For this review, take the finished solid that the model builds, in its own axes (mm). A direction names the side the tool comes from. Give positions to 0.01 mm unless a question says otherwise; leave off trailing zeros. Order: outer loops, then holes, each group sorted by start corner. A loop starts at its lowest first (then second) coordinate and runs counter-clockwise, first axis right, second up.
Autodesk Fusion 360 part; units mm, degrees
sketch "Sketch1" plane through (0, 0, 0) normal (0, 0, 1) x (1, 0, 0)
  line L0 (4, 0) -> (4, 18)
  line L1 (4, 18) -> (9, 18)
  line L2 (9, 18) -> (9, 39)
  line L3 (9, 39) -> (5, 39)
  line L4 (5, 39) -> (5, 22)
  line L5 (5, 22) -> (-5, 22)
  line L6 (-5, 22) -> (-5, 39)
  line L7 (-5, 39) -> (-9, 39)
  line L8 (-9, 39) -> (-9, 18)
  line L9 (-9, 18) -> (-4, 18)
  line L10 (-4, 18) -> (-4, 0)
  line L11 (-4, 0) -> (4, 0)
  point P0 (0, 22)
  dimension "d1" = 10
  dimension "d2" = 17
  dimension "d3" = 4
  dimension "d4" = 18
  dimension "d5" = 4
  dimension "d6" = 8
extrude "Extrude1" add sketch "Sketch1" along normal blind 15
sketch "Sketch2" plane through (-9, 0, 0) normal (-1, 0, 0) x (0, -1, 0)
  line L0 (-39, 0) -> (-18, 0)
  line L1 (-18, 0) -> (-18, 15)
  line L2 (-18, 15) -> (-39, 15)
  line L3 (-39, 15) -> (-39, 0)
  circle A0 centre (-32, 7.5) radius 1.6
  line L4 (-22, 0) -> (-22, 15)
  line L5 (-8.8, 11.1) -> (-5, 11.1)
  line L6 (-5, 11.1) -> (-5, 3.9)
  line L7 (-5, 3.9) -> (-8.8, 3.9)
  line L8 (-8.8, 3.9) -> (-8.8, 11.1)
  line L9 (-8.8, 11.1) -> (-5, 3.9) construction
  line L10 (-5, 11.1) -> (-8.8, 3.9) construction
  line L11 (0, 0) -> (0, 15)
  point P0 (-39, 7.5)
  point P1 (-6.9, 7.5)
  point P2 (0, 7.5)
  dimension "d9" = 3.2
  dimension "d11" = 10
  dimension "d18" = 7.2
  dimension "d19" = 3.8
  dimension "d20" = 5
extrude "Extrude2" cut sketch "Sketch2" against normal up to surface (18 mm away) contours A0 | L5 L6 L7 L8
ref_plane "WorkPlane1" through (0, 19.5, 7.5) normal (0, 0, 1) x (1, 0, 0)
sketch "Sketch4" plane through (0, 17, 7.5) normal (0, 0, 1) x (1, 0, 0)
  line L0 (-5, 16.6) -> (-5, 13.4)
  line L1 (-9, 13.4) -> (-9, 16.6)
  line L2 (9, 16.6) -> (9, 13.4)
  line L3 (5, 13.4) -> (5, 16.6)
  line L4 (-9, 15) -> (9, 15) construction
  line L5 (-5, 13.4) -> (-5, 11.9)
  line L6 (-5, 11.9) -> (-4.25, 12.9)
  line L7 (-4.25, 12.9) -> (-4.25, 13.4)
  line L8 (-4.25, 13.4) -> (-5, 13.4)
  line L9 (5, 13.4) -> (5, 11.9)
  line L10 (5, 11.9) -> (4.25, 12.9)
  line L11 (4.25, 12.9) -> (4.25, 13.4)
  line L12 (4.25, 13.4) -> (5, 13.4)
  dimension "d14" = 0.75
  dimension "d15" = 0.5
  dimension "d16" = 1.5
revolve "Revolve1" add sketch "Sketch4" angle 360 about axis through (-9, 32, 7.5) along (1, 0, 0)
sketch "Sketch5" plane through (0, 0, 0) normal (0, -1, 0) x (1, 0, 0)
  line L0 (-4, 0) -> (4, 0)
  line L1 (4, 0) -> (4, 15)
  line L2 (4, 15) -> (-4, 15)
  line L3 (-4, 15) -> (-4, 0)
  circle A0 centre (0, 7.5) radius 2.1
  point P0 (-4, 7.5)
  dimension "d21" = 4.2
extrude "Extrude3" cut sketch "Sketch5" against normal blind 19 contours A0
fillet "Fillet1" radius 3 4 edges at (-9, 18, 7.5) (-9, 39, 7.5) (9, 39, 7.5) (9, 18, 7.5)
chamfer "Chamfer1" distance 1 angle 45 4 edges at (0, 0, 15) (-4, 0, 7.5) (0, 0, 0) (4, 0, 7.5)
sketch "Sketch6" plane through (-9, 0, 0) normal (-1, 0, 0) x (0, -1, 0)
  circle A0 centre (-32, 7.5) radius 1.6
  line L0 (-36, 15) -> (-36, 0)
  line L1 (-36, 0) -> (-21, 0)
  line L2 (-21, 0) -> (-21, 15)
  line L3 (-21, 15) -> (-36, 15)
  line L4 (-33.6454, 10.35) -> (-35.2909, 7.5)
  line L5 (-35.2909, 7.5) -> (-33.6454, 4.65)
  line L6 (-33.6454, 4.65) -> (-30.3546, 4.65)
  line L7 (-30.3546, 4.65) -> (-28.7091, 7.5)
  line L8 (-28.7091, 7.5) -> (-30.3546, 10.35)
  line L9 (-30.3546, 10.35) -> (-33.6454, 10.35)
  point P0 (-32, 7.5)
  dimension "d50" = 5.7
extrude "Extrude4" cut sketch "Sketch6" against normal blind 2 contours L4 L5 L6 L7 L8 L9
sketch "Sketch7" plane through (9, 0, 0) normal (1, 0, 0) x (0, 1, 0)
  circle A0 centre (32, 7.5) radius 1.6
  line L0 (21, 15) -> (21, 0)
  line L1 (21, 0) -> (36, 0)
  line L2 (36, 0) -> (36, 15)
  line L3 (36, 15) -> (21, 15)
  circle A1 centre (32, 7.5) radius 3
  dimension "d53" = 6
extrude "Extrude5" cut sketch "Sketch7" against normal blind 2 contours A1
1) Draft analysis for pull direction Y (two halves, no side actions). For faces 1 (the face through (0, 7, 11.1)), 2 (the face through (-9, 27, 7)), 3 (the face through (-2, 0, 6)), state which applies: +Y half, -Y half, draft (parallel to the pull), parting line (faces both ways), or undercut.
Answer sheet:
face 1: undercut
face 2: draft
face 3: -Y half
2) Tool access review of faces 4 (the face through (-4, 10, 7)), 5 (the face through (-8, 32, 10.35)), 6 (the face through (-2, 8.8, 9)), 7 (the face through (-0.273, 2.465, 9.582)): name each direction out of +Z, -Z, +X, -X, +Y, -Y from which nothing blocks a thin tool from reaching the whole face with its end or side.
Answer sheet:
face 4: +Z, -Z, -X, -Y
face 5: -X
face 6: +X, -X
face 7: -Y
3) We need section A-A on y = 32. Count the separate pieces of the cut face and the enclosed holes in it, then the cut area to 3 significant figures.
Answer sheet:
separate pieces: 4
enclosed holes: 0
area: 86.8 mm2
4) Clearance check with flat-ended pins moving along their axes: pin 1 (3.5 mm diameter, centred on y = 32.5, z = 7.5, fed in from -X); pin 2 (3 mm diameter, centred on x = -2.5, z = 7.5, fed in from +Y); pin 3 (3 mm diameter, centred on y = 12.5, z = 10, fed in from -X). State where each tip first meets the part, or that it passes through.
Answer sheet:
pin 1: stops at x = -7
pin 2: stops at y = 22
pin 3: stops at x = -4
5) We need section B-B on y = 26.5. Give the boundary of the cut face in (x, z), then the cut area to 3 significant figures.
Answer sheet:
outline: (-9, 0) - (-5, 0) - (-5, 15) - (-9, 15) - close; (5, 0) - (9, 0) - (9, 15) - (5, 15) - close
area: 120 mm2
6) We need section D-D on x = 5.5. Give the boundary of the cut face in (y, z), then the cut area to 3 significant figures.
Answer sheet:
outline: (18, 0) - (39, 0) - (39, 15) - (18, 15) - close; hole circle Ø3.2 at (32, 7.5)
area: 307 mm2
7) We need section C-C on z = 3. Give the boundary of the cut face in (x, y), then the cut area to 3 significant figures.
Answer sheet:
outline: (-9, 21) arc R3 ccw to (-6, 18) - (-4, 18) - (-4, 1) - (-3, 0) - (3, 0) - (4, 1) - (4, 18) - (6, 18) arc R3 ccw to (9, 21) - (9, 36) arc R3 ccw to (6, 39) - (5, 39) - (5, 22) - (-5, 22) - (-5, 39) - (-6, 39) arc R3 ccw to (-9, 36) - close
area: 343 mm2
8) To check wall thickness, follow line 1 (Z direction, x = -2.75, y = 7.5); line 2 (Z direction, x = 6.2, y = 32); line 3 (X direction, y = 27, z = 8.75). State the ranges of each line that lie inside material, in increasing order.
Answer sheet:
line 1: z = 0 to 3.9, 11.1 to 15
line 2: z = 0 to 5.9, 9.1 to 15
line 3: x = -9 to -5, 5 to 9
